Geometry check sheet. Reference: the model listing, model coordinates, mm. A direction names the side the tool comes from. Give positions to 0.01 mm unless a question says otherwise; leave off trailing zeros. Order: outer loops, then holes, each group sorted by start corner. A loop starts at its lowest first (then second) coordinate and runs counter-clockwise, first axis right, second up. Notation, with made-up numbers: (68, 42.25) - (99, 42.25) arc R14 cw to (99, 68.25) - close; hole circle Ø7 at (9, 35.5). An arc over 180 degrees is marked (long way). Put each result on its own line as item: value. Start each with the question number.
```python
from build123d import *

# Parameters (mm, degrees)
F0_W     = 114.3
F0_H     = 88.9
F1_DEPTH = 152.4
F2_W     = 25.4
F2_H     = 88.9
F3_DEPTH = 88.901
F4_R     = 38.1
F5_R     = 12.7
F6_DEPTH = 114.301
F7_R     = 6.35
F8_DEPTH = 38.1


with BuildPart() as f1:
    # F0 (on Top) → F1 (new body)
    with BuildSketch(Plane.XY):
        Rectangle(F0_W, F0_H)
    extrude(amount=F1_DEPTH)

    # F2 (on face) → F3 (cut, through all)
    with BuildSketch(Plane.XZ.offset(44.45)):
        with Locations((-25.4, 107.95)):
            Rectangle(F2_W, F2_H)
        with Locations((25.4, 107.95)):
            Rectangle(F2_W, F2_H)
    extrude(amount=-F3_DEPTH, mode=Mode.SUBTRACT)

    # F4
    f4_edges = [f1.edges().sort_by_distance(p)[0] for p in [
        (47.625, -44.45, 152.4),
        (0, -44.45, 152.4),
        (-47.625, -44.45, 152.4),
        (-47.625, 44.45, 152.4),
        (0, 44.45, 152.4),
        (47.625, 44.45, 152.4),
    ]]
    fillet(f4_edges, radius=F4_R)

    # F5 (on face) → F6 (cut, through all)
    with BuildSketch(Plane(origin=(-57.15, 0, 0), x_dir=(0, -1, 0), z_dir=(-1, 0, 0))):
        with Locations((0, 38.1)):
            Circle(F5_R)
        with Locations((0, 114.3)):
            Circle(F5_R)
    extrude(amount=-F6_DEPTH, mode=Mode.SUBTRACT)

    # F7 (on face) → F8 (cut)
    with BuildSketch(Plane(origin=(0, 0, 0), x_dir=(1, 0, 0), z_dir=(0, 0, -1))):
        Circle(F7_R)
    extrude(amount=-F8_DEPTH, mode=Mode.SUBTRACT)


solid = f1.part
```
Item 1: Cross-section at D-D (z = 70). Enter the section's corners in (x, y), and give its area (3 significant figures).
Item 2: Cross-section at A-A (y = 0). Count the separate pieces of the cut face and the enclosed holes in it, and give its area (3 significant figures).
Item 3: Cross-section at B-B (z = 38.1). Enter the section's corners in (x, y), and give its area (3 significant figures).
Item 4: Set-up check for faces 3 (the face through (47.76, 33.59, 140.94)), 4 (the face through (-12.7, -1, 97)): record each of +Z, -Z, +X, -X, +Y, -Y from which the full face is reachable in a straight line by a thin tool's end or side.
Item 5: Gauge pin test, flat ends, axial feed: pin 1 Ø12 at (y, z) = (0.5, 40.5) entering from -X; pin 2 Ø12 at (x, z) = (-16, 128) entering from -Y; pin 3 Ø6 at (x, y) = (-24.5, -35) entering from +Z; pin 4 Ø7.5 at (x, y) = (0, 0) entering from -Z. Record the tip position at first contact, or that the pin passes through.
Item 6: Thickness scan on line 1 along X through (y, z) = (-23.5, 144.5); line 2 along Z through (x, y) = (12.5, 0). Record the ranges inside material, lowest first.
Item 7: Release check for a two-part mould opening along X. For faces 1 (the face through (6.057, -1.907, 13.361)), 2 (the face through (-1, -44.45, 44)) record: +X half, -X half, draft (parallel to the pull), parting line (faces both ways), or undercut.
Item 8: Cross-section at C-C (x = 0). Enter the section's corners in (y, z), and give its area (3 significant figures).
Recorded:
1. outline: (-57.15, -44.45) - (-38.1, -44.45) - (-38.1, 44.45) - (-57.15, 44.45) - close; (-12.7, -44.45) - (12.7, -44.45) - (12.7, 44.45) - (-12.7, 44.45) - close; (38.1, -44.45) - (57.15, -44.45) - (57.15, 44.45) - (38.1, 44.45) - close
1. area: 5,650 mm^2
2. separate pieces: 6
2. enclosed holes: 0
2. area: 8,060 mm^2
3. outline: (-57.15, -44.45) - (57.15, -44.45) - (57.15, -12.7) - (-57.15, -12.7) - close; (-57.15, 12.7) - (57.15, 12.7) - (57.15, 44.45) - (-57.15, 44.45) - close
3. area: 7,260 mm^2
4. face 3: +Z, +X, -X, +Y
4. face 4: +Z, +Y, -Y
5. pin 1: passes through
5. pin 2: stops at y = -43.45
5. pin 3: stops at z = 63.5
5. pin 4: stops at z = 50.23
6. line 1: x = -57.15 to -38.1, -12.7 to 12.7, 38.1 to 57.15
6. line 2: z = 0 to 25.4, 50.8 to 101.6, 127 to 152.4
7. face 1: undercut
7. face 2: draft
8. outline: (-44.45, 0) - (-6.35, 0) - (-6.35, 27.1) arc R12.7 cw (long way) to (6.35, 27.1) - (6.35, 0) - (44.45, 0) - (44.45, 114.3) arc R38.1 ccw to (6.35, 152.4) - (-6.35, 152.4) arc R38.1 ccw to (-44.45, 114.3) - close; hole circle Ø25.4 at (0, 114.3)
8. area: 11,600 mm^2
